```python
from build123d import *

# Parameters (mm, degrees)
SKETCH1_W                = 60
SKETCH1_H                = 84
BOSS_EXTRUDE2_DEPTH      = 82
BOSS_EXTRUDE2_DEPTH_BACK = 25
SKETCH2_W                = 56
SKETCH2_H                = 80
CUT_EXTRUDE1_DEPTH       = 108
BOSS_EXTRUDE6_DEPTH      = 107
SKETCH22_R               = 1.95
CUT_EXTRUDE6_DEPTH       = 25
CUT_EXTRUDE9_DEPTH       = 2
SKETCH28_W               = 8
SKETCH28_H               = 85.946450773
CUT_EXTRUDE11_DEPTH      = 60
BOSS_EXTRUDE9_DEPTH      = 84
SKETCH37_R               = 1.6
CUT_EXTRUDE15_DEPTH      = 4
CUT_EXTRUDE16_DEPTH      = 4
SKETCH41_R               = 2
CUT_EXTRUDE17_DEPTH      = 2
SKETCH42_R               = 11.5
CUT_EXTRUDE18_DEPTH      = 2.5
SKETCH43_R               = 5
CUT_EXTRUDE19_DEPTH      = 1.5
SKETCH44_R               = 3
CUT_EXTRUDE20_DEPTH      = 2


with BuildPart() as part:
    # Sketch1 → Boss-Extrude2 (new body, two sides)
    with BuildSketch(Plane.XY) as boss_extrude2_sk:
        with Locations((30, 42)):
            Rectangle(SKETCH1_W, SKETCH1_H)
    extrude(amount=BOSS_EXTRUDE2_DEPTH)
    extrude(boss_extrude2_sk.sketch, amount=-BOSS_EXTRUDE2_DEPTH_BACK)

    # Sketch2 → Cut-Extrude1 (cut, through all)
    with BuildSketch(Plane.XY.offset(82)):
        with Locations((30, 42)):
            Rectangle(SKETCH2_W, SKETCH2_H)
    extrude(amount=-CUT_EXTRUDE1_DEPTH, mode=Mode.SUBTRACT)

    # Sketch8 → Boss-Extrude6 (add)
    with BuildSketch(Plane(origin=(0, 0, -25), x_dir=(-1, 0, 0), z_dir=(0, 0, -1))):
        with BuildLine():
            Line((-58, 82), (-52, 82))
            Line((-52, 82), (-52, 78))
            ThreePointArc((-52, 78), (-52.585786438, 76.585786438), (-54, 76))
            Line((-54, 76), (-58, 76))
            Line((-58, 76), (-58, 82))
        make_face()
        with BuildLine():
            Line((-2, 2), (-8, 2))
            Line((-8, 2), (-8, 6))
            ThreePointArc((-8, 6), (-7.414213562, 7.414213562), (-6, 8))
            Line((-6, 8), (-2, 8))
            Line((-2, 8), (-2, 2))
        make_face()
        with BuildLine():
            Line((-2, 76), (-2, 82))
            Line((-2, 82), (-8, 82))
            Line((-8, 82), (-8, 78))
            ThreePointArc((-8, 78), (-7.414213562, 76.585786438), (-6, 76))
            Line((-6, 76), (-2, 76))
        make_face()
        with BuildLine():
            Line((-58, 8), (-58, 2))
            Line((-58, 2), (-52, 2))
            Line((-52, 2), (-52, 6))
            ThreePointArc((-52, 6), (-52.585786438, 7.414213562), (-54, 8))
            Line((-54, 8), (-58, 8))
        make_face()
    extrude(amount=-BOSS_EXTRUDE6_DEPTH)

    # Sketch22 → Cut-Extrude6 (cut)
    with BuildSketch(Plane(origin=(0, 0, -25), x_dir=(-1, 0, 0), z_dir=(0, 0, -1))):
        with Locations((-56, 80)):
            Circle(SKETCH22_R)
        with Locations((-4, 80)):
            Circle(SKETCH22_R)
        with Locations((-4, 4)):
            Circle(SKETCH22_R)
        with Locations((-56, 4)):
            Circle(SKETCH22_R)
    cut_extrude6 = extrude(amount=-CUT_EXTRUDE6_DEPTH, mode=Mode.SUBTRACT)

    # Sketch26 → Cut-Extrude9 (cut)
    with BuildSketch(Plane(origin=(0, 84, 0), x_dir=(1, 0, 0), z_dir=(0, 1, 0))):
        Polygon((15, -57), (10.8, -57), (10.8, -47), (19.2, -47), (19.2, -57), align=None)
        Polygon((40.8, -47), (40.8, -57), (45, -57), (49.2, -57), (49.2, -47), align=None)
    extrude(amount=-CUT_EXTRUDE9_DEPTH, mode=Mode.SUBTRACT)

    # Sketch28 → Cut-Extrude11 (cut)
    with BuildSketch(Plane.ZY):
        with Locations((78, 41.026774614)):
            Rectangle(SKETCH28_W, SKETCH28_H)
    extrude(amount=-CUT_EXTRUDE11_DEPTH, mode=Mode.SUBTRACT)

    # Sketch32 → Boss-Extrude9 (add)
    with BuildSketch(Plane(origin=(0, 84, 0), x_dir=(1, 0, 0), z_dir=(0, 1, 0))):
        Polygon((60, -33), (60, -35), (0, -35), (0, -33), (0, -31), (60, -31), align=None)
    extrude(amount=-BOSS_EXTRUDE9_DEPTH)

    # Sketch37 → Cut-Extrude15 (cut)
    with BuildSketch(Plane(origin=(0, 0, 31), x_dir=(-1, 0, 0), z_dir=(0, 0, -1))):
        with Locations((-15, 57)):
            Circle(SKETCH37_R)
        with Locations((-45, 57)):
            Circle(SKETCH37_R)
        with Locations((-45, 27)):
            Circle(SKETCH37_R)
        with Locations((-15, 27)):
            Circle(SKETCH37_R)
    extrude(amount=-CUT_EXTRUDE15_DEPTH, mode=Mode.SUBTRACT)

    # Sketch38 → Cut-Extrude16 (cut)
    with BuildSketch(Plane(origin=(0, 0, 31), x_dir=(-1, 0, 0), z_dir=(0, 0, -1))):
        Polygon((-30, 7), (-45, 7), (-45, 17), (-15, 17), (-15, 7), align=None)
    extrude(amount=-CUT_EXTRUDE16_DEPTH, mode=Mode.SUBTRACT)

    # Mirror1: Cut-Extrude6 across plane
    add(cut_extrude6.mirror(Plane(origin=(0, 0, 24.5), x_dir=(1, 0, 0), z_dir=(0, 0, -1))), mode=Mode.SUBTRACT)

    # Sketch41 → Cut-Extrude17 (cut)
    with BuildSketch(Plane(origin=(0, 84, 0), x_dir=(1, 0, 0), z_dir=(0, 1, 0))):
        with Locations((30, -63)):
            Circle(SKETCH41_R)
    extrude(amount=-CUT_EXTRUDE17_DEPTH, mode=Mode.SUBTRACT)

    # Sketch42 → Cut-Extrude18 (cut)
    with BuildSketch(Plane(origin=(0, 0, 31), x_dir=(-1, 0, 0), z_dir=(0, 0, -1))):
        with Locations((-30, 42)):
            Circle(SKETCH42_R)
    extrude(amount=-CUT_EXTRUDE18_DEPTH, mode=Mode.SUBTRACT)

    # Sketch43 → Cut-Extrude19 (cut)
    with BuildSketch(Plane(origin=(0, 0, 33.5), x_dir=(-1, 0, 0), z_dir=(0, 0, -1))):
        with Locations((-30, 42)):
            Circle(SKETCH43_R)
    extrude(amount=-CUT_EXTRUDE19_DEPTH, mode=Mode.SUBTRACT)

    # Sketch44 → Cut-Extrude20 (cut)
    with BuildSketch(Plane.XZ):
        with Locations((20, 64)):
            Circle(SKETCH44_R)
        with Locations((40, 64)):
            Circle(SKETCH44_R)
        Polygon((30, 69.5), (25.5, 69.5), (25.5, 60.5), (34.5, 60.5), (34.5, 69.5), align=None)
    extrude(amount=-CUT_EXTRUDE20_DEPTH, mode=Mode.SUBTRACT)


solid = part.part
```
Geometry check sheet. Reference: the model listing, model coordinates, mm. A direction names the side the tool comes from. Round coordinates to 2 decimals unless told otherwise and drop trailing zeros. Order: outer loops, then holes, each group sorted by start corner. A loop starts at its lowest first (then second) coordinate and runs counter-clockwise, first axis right, second up. Notation, with made-up numbers: (16.5, 88.25) - (55.5, 88.25) arc R16 cw to (55.5, 100.25) - close; hole circle Ø4 at (73.25, 47). An arc over 180 degrees is marked (long way). Use a Markdown table: item, result. Add a question column.
(1) Sectioned sample at B-B, the plane y = 42. Enter the section's corners in (x, z).
(2) Depth check by flat-ended pin: pin 1 (2.5 mm diameter, centred on x = 4, y = 80, fed in from +Z); pin 2 (5 mm diameter, centred on x = 7.5, y = 60, fed in from +Z); pin 3 (8 mm diameter, centred on x = 53.5, y = 13.5, fed in from -Z). Enter the tip coordinate at first touch or a pass-through.
(3) Material ranges on line 1 along X through (y, z) = (63, -19); line 2 along Y through (x, z) = (16, 3.5); line 3 along Y through (x, z) = (56, -16.75), recorded low to high. Write a range as [from, to].
(4) Release check for a two-part mould opening along Y. For faces 4 (the cylindrical face through (31.075, 83.014, 61.314)), 5 (the flat face through (4, 4, 0)), 6 (the flat face through (30, 82, 55)) record: pulls with the +Y half, pulls with the -Y half, needs draft (parallel to the pull), parting line crosses it, or undercut.
(5) Sectioned sample at A-A, the plane z = 50.5. Count the separate pieces of the cut face and the enclosed holes in it, and give its area (3 significant figures).
(6) Sectioned sample at C-C, the plane z = -16.5. Enter the section's corners in (x, y).
(7) Tool access check on faces 1 (the flat face through (45, 12, 33)), 2 (the cylindrical face through (54.14, 80.59, 61.68)), 3 (the flat face through (4, 8, 3)). Record the directions out of +Z, -Z, +X, -X, +Y, -Y that give a thin tool (end or side, any length) a straight path to the whole face; none if there is none.
Answers below:
| question | item | result |
|---|---|---|
| 1 | outline | (0, -25) - (2, -25) - (2, 31) - (18.5, 31) - (18.5, 33.5) - (25, 33.5) - (25, 35) - (2, 35) - (2, 74) - (0, 74) - close; (35, 33.5) - (41.5, 33.5) - (41.5, 31) - (58, 31) - (58, -25) - (60, -25) - (60, 74) - (58, 74) - (58, 35) - (35, 35) - close |
| 2 | pin 1 | z = 49 |
| 2 | pin 2 | z = 35 |
| 2 | pin 3 | z = 31 |
| 3 | line 1 | [0, 2], [58, 60] |
| 3 | line 2 | [0, 2], [82, 84] |
| 3 | line 3 | [0, 2.05], [5.95, 8], [76, 78.05], [81.95, 84] |
| 4 | face 4 | needs draft |
| 4 | face 5 | undercut |
| 4 | face 6 | undercut |
| 5 | separate pieces | 2 |
| 5 | enclosed holes | 4 |
| 5 | area | 619 mm² |
| 6 | outline | (0, 0) - (60, 0) - (60, 84) - (0, 84) - close; hole (2, 8) - (6, 8) arc R2 cw to (8, 6) - (8, 2) - (52, 2) - (52, 6) arc R2 cw to (54, 8) - (58, 8) - (58, 76) - (54, 76) arc R2 cw to (52, 78) - (52, 82) - (8, 82) - (8, 78) arc R2 cw to (6, 76) - (2, 76) - close; hole circle Ø3.9 at (4, 4); hole circle Ø3.9 at (4, 80); hole circle Ø3.9 at (56, 4); hole circle Ø3.9 at (56, 80) |
| 7 | face 1 | +Z, -Z |
| 7 | face 2 | +Z |
| 7 | face 3 | -Z |
